from build123d import *

# Parameters (mm, degrees)
SKETCH_1_W               = 93
SKETCH_1_H               = 48
EXTRUDE_1_DEPTH          = 3
SKETCH_2_R               = 2.7
SKETCH_2_R_2             = 1.6
CUT_EXTRUDE_1_DEPTH      = 53.414215629
PATTERN_CIRCULAR_1_COUNT = 4
SKETCH_3_W               = 28
SKETCH_3_H               = 26
CUT_EXTRUDE_2_DEPTH      = 53.414215629
FILLET_1_R               = 1
CHAMFER_1_SIZE           = 3


with BuildPart() as part:
    # 草圖1 → 填料-伸長1 (new body)
    with BuildSketch(Plane.XY):
        Rectangle(SKETCH_1_W, SKETCH_1_H)
    extrude(amount=EXTRUDE_1_DEPTH)

    # 草圖2 → 除料-伸長1 (cut, through all)
    with BuildSketch(Plane.XY.offset(3)):
        with Locations((-35.5, 13)):
            Circle(SKETCH_2_R)
        with Locations((-28.5, 13)):
            Circle(SKETCH_2_R_2)
    cut_extrude_1 = extrude(amount=-CUT_EXTRUDE_1_DEPTH, mode=Mode.SUBTRACT)

    # 環狀複製排列1: 除料-伸長1 ×4 about axis
    pattern_circular_1_axis = Axis((-35.5, 13, 0), (0, 0, 1))
    for i in range(1, PATTERN_CIRCULAR_1_COUNT):
        add(cut_extrude_1.rotate(pattern_circular_1_axis, i * 360 / PATTERN_CIRCULAR_1_COUNT), mode=Mode.SUBTRACT)

    # 草圖3 → 除料-伸長2 (cut, through all)
    with BuildSketch(Plane.XY.offset(3)):
        with Locations((-32.5, -11)):
            Rectangle(SKETCH_3_W, SKETCH_3_H)
    extrude(amount=-CUT_EXTRUDE_2_DEPTH, mode=Mode.SUBTRACT)

    # 圓角1
    fillet_1_edges = [part.edges().sort_by_distance(p)[0] for p in [
        (-18.5, 2, 1.5),
    ]]
    fillet(fillet_1_edges, radius=FILLET_1_R)

    # 導角1
    chamfer_1_edges = [part.edges().sort_by_distance(p)[0] for p in [
        (-46.5, 2, 1.5),
        (-18.5, -24, 1.5),
        (-46.5, 24, 1.5),
        (46.5, 24, 1.5),
        (46.5, -24, 1.5),
    ]]
    chamfer(chamfer_1_edges, length=CHAMFER_1_SIZE)


solid = part.part
For this review, take the finished solid that the model builds, in its own axes (mm). A direction names the side the tool comes from. Give positions to 0.01 mm unless a question says otherwise; leave off trailing zeros. Order: outer loops, then holes, each group sorted by start corner. A loop starts at its lowest first (then second) coordinate and runs counter-clockwise, first axis right, second up. Notation, with made-up numbers: M -8,26 L 21,26 A10 cw 21,35 Z; hole C 75,-33 d3. An arc over 180 degrees is marked long. Answer in a Markdown table with one row per item. Add a question column.
(1) Mouldability with a two-part tool opening along X and no side actions: class faces 3 (the face through (45, 22.5, 1.5)), 4 (the face through (-29.68, 14.08, 1.52)), 5 (the face through (10, 0, 3)) as +X half, -X half, draft (parallel to the pull), parting line (faces both ways), or undercut.
(2) Consider section B-B on x = -42.5. State the section outline as (y, z) points, and give its area (3 significant figures).
(3) Consider section C-C on y = 6. State the section outline as (x, z) points.
(4) Consider section D-D on x = -20.5. State the section outline as (y, z) points.
(5) For faces 1 (the face through (-36.92, 5.26, 1.52)), 2 (the face through (-32, 2, 2)), list the 3-axis set-ups (+Z, -Z, +X, -X, +Y, -Y) from which the entire face can be reached by the end or side of a thin tool; tool diameter is ignored.
(6) Consider section A-A on y = 13. State the section outline as (x, z) points.
(7) Wall thickness on probe 1 along Y at (x, z) = (-42.5, 1.1); probe 2 along X at (y, z) = (6, 1.1); probe 3 along X at (y, z) = (-17, 0.3): over which ranges is each line inside the solid? List them lowest first. Write a range as [from, to].
(8) For pin 1 (1.5 mm diameter, centred on x = -30, z = 1.5, fed in from -Y); pin 2 (1.5 mm diameter, centred on y = -19, z = 1, fed in from -X), all flat-tipped, find the tip position at first contact; note any pin that passes through.
Evaluation:
| question | item | result |
|---|---|---|
| 1 | face 3 | +X half |
| 1 | face 4 | undercut |
| 1 | face 5 | draft |
| 2 | outline | M 2,0 L 11.4,0 L 11.4,3 L 2,3 Z; M 14.6,0 L 24,0 L 24,3 L 14.6,3 Z |
| 2 | area | 56.4 mm^2 |
| 3 | outline | M -46.5,0 L -37.1,0 L -37.1,3 L -46.5,3 Z; M -33.9,0 L 46.5,0 L 46.5,3 L -33.9,3 Z |
| 4 | outline | M 2,0 L 24,0 L 24,3 L 2,3 Z |
| 5 | face 1 | +Z, -Z |
| 5 | face 2 | +Z, -Z, -X, -Y |
| 6 | outline | M -46.5,0 L -44.1,0 L -44.1,3 L -46.5,3 Z; M -40.9,0 L -38.2,0 L -38.2,3 L -40.9,3 Z; M -32.8,0 L -30.1,0 L -30.1,3 L -32.8,3 Z; M -26.9,0 L 46.5,0 L 46.5,3 L -26.9,3 Z |
| 7 | probe 1 | y = [2, 11.4], [14.6, 24] |
| 7 | probe 2 | x = [-46.5, -37.1], [-33.9, 46.5] |
| 7 | probe 3 | x = [-18.5, 46.5] |
| 8 | pin 1 | stops at y = 2 |
| 8 | pin 2 | stops at x = -18.5 |
